```python
from build123d import *

# Parameters (mm, degrees)
EXTRUDE_1_DEPTH          = 10
SKETCH_2_R               = 3.75
CUT_EXTRUDE_2_DEPTH      = 21
CUT_EXTRUDE_2_DEPTH_BACK = 1
CUT_EXTRUDE_3_DEPTH      = 4
CUT_EXTRUDE_3_DEPTH_BACK = 4
CUT_EXTRUDE_4_DEPTH      = 12


with BuildPart() as part:
    # 草图1 → 凸台-拉伸1 (new body, symmetric)
    with BuildSketch(Plane(origin=(0, 0, 0), x_dir=(1, 0, 0), z_dir=(0, 1, 0))):
        with BuildLine():
            Line((-14.142135624, 14.142135624), (-63.639610307, -35.355339059))
            ThreePointArc((-63.639610307, -35.355339059), (-109.455133557, -88.069120133), (-147.47848225, -146.652648876))
            ThreePointArc((-147.47848225, -146.652648876), (-122.47848225, -171.652648876), (-97.47848225, -146.652648876))
            ThreePointArc((-97.47848225, -146.652648876), (-84.10519624, -105.787977439), (-56.088247687, -73.171773734))
            Line((-56.088247687, -73.171773734), (12.855752194, -15.320888862))
            ThreePointArc((12.855752194, -15.320888862), (14.745546736, 13.511804152), (-14.142135624, 14.142135624))
        make_face()
    extrude(amount=EXTRUDE_1_DEPTH, both=True)

    # 草图2 → 切除-拉伸2 (cut, two sides)
    with BuildSketch(Plane(origin=(0, 10, 0), x_dir=(-1, 0, 0), z_dir=(0, -1, 0))) as cut_extrude_2_sk:
        Circle(SKETCH_2_R)
    extrude(amount=CUT_EXTRUDE_2_DEPTH, mode=Mode.SUBTRACT)
    extrude(cut_extrude_2_sk.sketch, amount=-CUT_EXTRUDE_2_DEPTH_BACK, mode=Mode.SUBTRACT)

    # 草图3 → 切除-拉伸3 (cut, two sides)
    with BuildSketch(Plane(origin=(0, 10, 0), x_dir=(-1, 0, 0), z_dir=(0, -1, 0))) as cut_extrude_3_sk:
        with BuildLine():
            add(Edge.make_bspline(
                [(-3.457188478, 3.680182522), (-18, 3.087230439), (-18, 0), (-18, -3.087230439), (-3.457188478, -3.680182522)],
                knots=[1.764063263, 1.764063263, 1.764063263, 3.141592654, 3.141592654, 4.519122044, 4.519122044, 4.519122044], degree=2, weights=[1, 0.772031744, 1, 0.772031744, 1]))
            add(Edge.make_bspline(
                [(-3.457188478, -3.680182522), (0, -24.523240209), (3.457188478, -3.680182522)],
                knots=[1.968592603, 1.968592603, 1.968592603, 4.314592705, 4.314592705, 4.314592705], degree=2, weights=[1, 0.387387634, 1]))
            add(Edge.make_bspline(
                [(3.457188478, -3.680182522), (18, -3.087230439), (18, 0), (18, 3.087230439), (3.457188478, 3.680182522)],
                knots=[4.905655917, 4.905655917, 4.905655917, 6.283185307, 6.283185307, 7.660714698, 7.660714698, 7.660714698], degree=2, weights=[1, 0.772031744, 1, 0.772031744, 1]))
            add(Edge.make_bspline(
                [(3.457188478, 3.680182522), (0, 24.523240209), (-3.457188478, 3.680182522)],
                knots=[5.110185256, 5.110185256, 5.110185256, 7.456185358, 7.456185358, 7.456185358], degree=2, weights=[1, 0.387387634, 1]))
        make_face()
    extrude(amount=CUT_EXTRUDE_3_DEPTH, mode=Mode.SUBTRACT)
    extrude(cut_extrude_3_sk.sketch, amount=-CUT_EXTRUDE_3_DEPTH_BACK, mode=Mode.SUBTRACT)

    # 草图4 → 切除-拉伸4 (cut)
    with BuildSketch(Plane(origin=(0, -10, 0), x_dir=(-1, 0, 0), z_dir=(0, -1, 0))):
        with BuildLine():
            Line((0, -26.108145787), (54.796803902, -26.512532655))
            Line((54.796803902, -26.512532655), (14.772467095, 13.511804152))
            ThreePointArc((14.772467095, 13.511804152), (-14.441332679, 13.851832142), (-12.855752194, -15.320888862))
            Line((-12.855752194, -15.320888862), (0, -26.108145787))
        make_face()
    extrude(amount=-CUT_EXTRUDE_4_DEPTH, mode=Mode.SUBTRACT)


solid = part.part
```
Model file for the job. Use its own axes, mm. A direction names the side the tool comes from. Round coordinates to 2 decimals unless told otherwise and drop trailing zeros. Write each loop counter-clockwise with the first axis right and the second up, starting at its lowest first coordinate (ties: lowest second). Pieces come first, ordered by that corner, then holes. Notation, with made-up numbers: (-23.5, -25) - (4.5, -25) arc R22 cw to (4.5, 10) - close; hole circle Ø6 at (74.25, -8.5). An arc over 180 degrees is marked (long way). One line per item, written item: value.
(1) Cut at B-B, the plane x = -50.5. Give the cut face in (y, z).
Values follow:
outline: (-10, 26.48) - (2, 26.48) - (2, 22.22) - (10, 22.22) - (10, 68.48) - (-10, 68.48) - close
(2) Cut at D-D, the plane z = 156. Give the cut face in (x, y).
Values follow:
outline: (-145.67, -10) - (-99.29, -10) - (-99.29, 10) - (-145.67, 10) - close
(3) Cut at A-A, the plane y = -0.5. Give the cut face in (x, z).
Values follow:
outline: (-147.48, 146.65) arc R500 ccw to (-63.64, 35.36) - (-54.8, 26.51) - (0, 26.11) - (-56.09, 73.17) arc R110 cw to (-97.48, 146.65) arc R25 ccw to start
(4) Wall check: probe 1 along Z at (x, y) = (0, 2.9); probe 2 along Y at (x, z) = (9.5, -5); probe 3 along X at (y, z) = (4, 135). Give the ranges that are in metal, low to high.
Values follow:
probe 1: z = -20 to -3.75, 3.75 to 26.11
probe 2: y = 2 to 10
probe 3: x = -140.82 to -95.44
(5) 3-axis set-ups, long thin cutter, end or side, ignore diameter. For faces 1 (the flat face through (1, 6, 4)), 2 (the flat face through (-70, 10, 73)): which of +Z, -Z, +X, -X, +Y, -Y reach the whole face in a straight line?
Values follow:
face 1: +Y
face 2: +Z, -Z, +X, -X, +Y
(6) Two-plate mould, pull along X, no slides. Class faces 3 (the cylindrical face through (3.746, 4.028, -0.165)), 4 (the cylindrical face through (-84.401, 0.14, 106.317)), 5 (the cylindrical face through (-123.028, 0.14, 171.647)): pulls with the +X half, pulls with the -X half, needs draft (parallel to the pull), parting line crosses it, or undercut.
Values follow:
face 3: undercut
face 4: pulls with the +X half
face 5: parting line crosses it
(7) Drop flat-ended pins along their axis: P1, Ø10, axis at y = -4, z = 111.5, coming from the -X side; P2, Ø12, axis at x = -117.5, y = 1.5, coming from the -Z side; P3, Ø23.5, axis at x = -2.5, z = -3.5, coming from the -Y side. Give the stop position or say it passes through.
Values follow:
P1: stops at x = -129.36
P2: stops at z = 90.8
P3: stops at y = 2
(8) Cut at C-C, the plane z = 69. Give the cut face in (x, y), plus the area to 3 significant figures.
Values follow:
outline: (-94.35, -10) - (-51.12, -10) - (-51.12, 10) - (-94.35, 10) - close
area: 865 mm²
